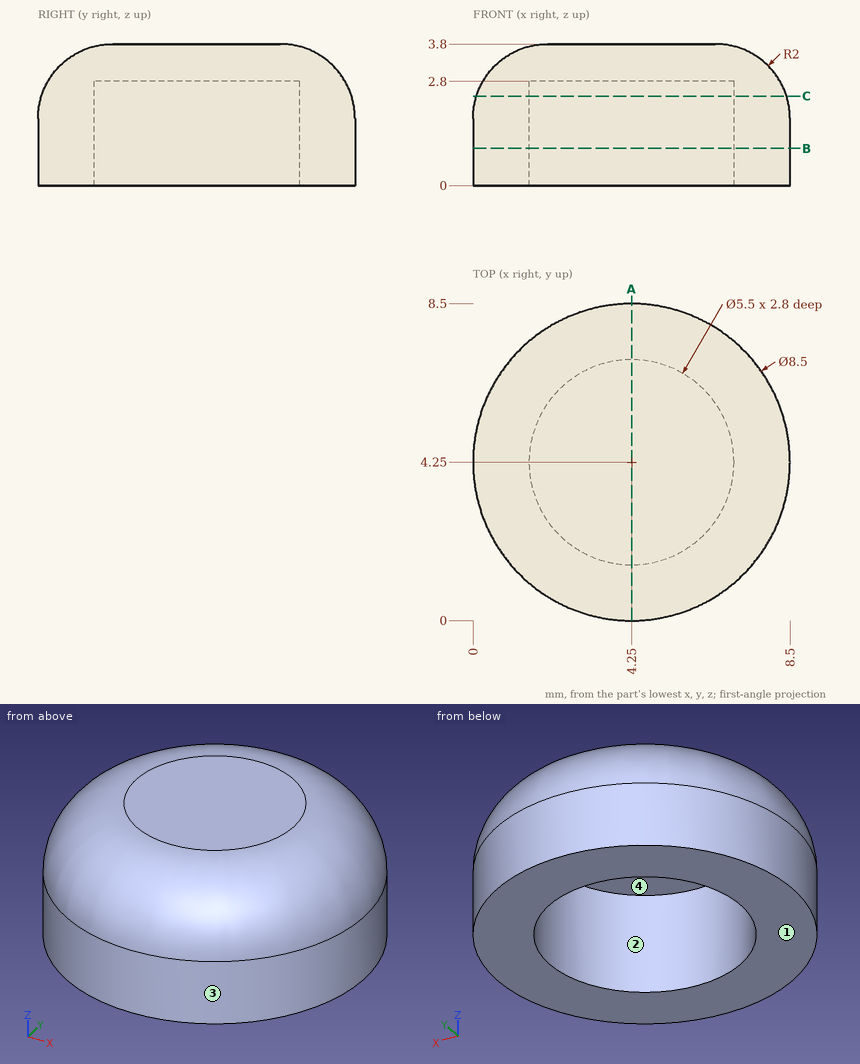
Part print with two shaded views. Sizes in mm from the minimum x, y, z corner. Round coordinates to 2 decimals unless told otherwise and drop trailing zeros. Order: outer loops, then holes, each group sorted by start corner. A loop starts at its lowest first (then second) coordinate and runs counter-clockwise, first axis right, second up.
(1) Band-saw the part on C-C (z = 2.4). List the corners of the cut face in (x, y), then the cut area to 3 significant figures.
(2) Band-saw the part on A-A (x = 4.25). List the corners of the cut face in (y, z), then the cut area to 3 significant figures.
(3) Pin check, flat tips, straight feed: pin 1 (1.5 mm diameter, centred on y = 6.5, z = 3, fed in from +X); pin 2 (2 mm diameter, centred on x = 2, y = 1, fed in from +Z); pin 3 (4.5 mm diameter, centred on x = 4, y = 4.5, fed in from -Z). Stop position of each tip, or through.
(4) Drill centre lines: line 1 (Y direction, x = 4.25, z = 0.7); line 2 (Z direction, x = 5.75, y = 4.25); line 3 (X direction, y = 5.5, z = 0.65). Where is each one in solid material? Low to high.
(5) Pull direction X, two halves, no side cores. Call the marked faces 1, 2, 3 and 4: released by +X, released by -X, zero draft, split by the parting line, or undercut.
(6) Band-saw the part on B-B (z = 1). List the corners of the cut face in (x, y), then the cut area to 3 significant figures.
Verdict:
1. outline: circle Ø8.32 at (4.25, 4.25); hole circle Ø5.5 at (4.25, 4.25)
1. area: 30.6 mm2
2. outline: (0, 0) - (1.5, 0) - (1.5, 2.8) - (7, 2.8) - (7, 0) - (8.5, 0) - (8.5, 1.8) arc R2 ccw to (6.5, 3.8) - (2, 3.8) arc R2 ccw to (0, 1.8) - close
2. area: 15.2 mm2
3. pin 1: stops at x = 8.01
3. pin 2: stops at z = 3.67
3. pin 3: stops at z = 2.8
4. line 1: y = 0 to 1.5, 7 to 8.5
4. line 2: z = 2.8 to 3.8
4. line 3: x = 0.19 to 1.8, 6.7 to 8.31
5. face 1: zero draft
5. face 2: undercut
5. face 3: split by the parting line
5. face 4: undercut
6. outline: circle Ø8.5 at (4.25, 4.25); hole circle Ø5.5 at (4.25, 4.25)
6. area: 33.0 mm2
